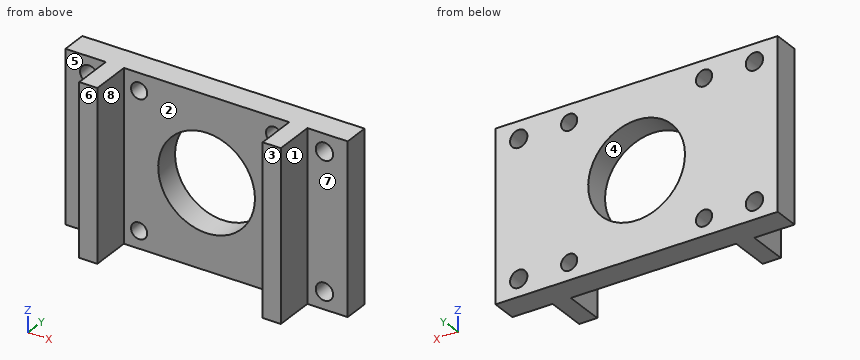
```python
from build123d import *

# Parameters (mm, degrees)
SKETCH1_W             = 70
SKETCH1_H             = 42
BOSS_EXTRUDE1_DEPTH   = 3.175
SKETCH3_W             = 4.5
SKETCH3_H             = 42
BOSS_EXTRUDE2_DEPTH   = 10
F_1_0MM_DOWEL_HOLE1_D = 4
F_1_0MM_DOWEL_HOLE2_D = 4.3
SKETCH4_R             = 12
CUT_EXTRUDE1_DEPTH    = 44.969563336


with BuildPart() as part:
    # Sketch1 → Boss-Extrude1 (new, symmetric)
    with BuildSketch(Plane(origin=(0, 0, 0), x_dir=(1, 0, 0), z_dir=(0, 1, 0))):
        Rectangle(SKETCH1_W, SKETCH1_H)
    extrude(amount=BOSS_EXTRUDE1_DEPTH, both=True)

    # Sketch3 → Boss-Extrude2 (add)
    with BuildSketch(Plane.XZ.offset(3.175)):
        with Locations((-22.75, 0)):
            Rectangle(SKETCH3_W, SKETCH3_H)
        with Locations((22.75, 0)):
            Rectangle(SKETCH3_W, SKETCH3_H)
    extrude(amount=BOSS_EXTRUDE2_DEPTH)

    # Ø1.0mm Dowel Hole1 (through all)
    with Locations(Plane(origin=(0, 3.175, 0), x_dir=(1, 0, 0), z_dir=(0, 1, 0))):
        with Locations((-16.73, 16.73), (16.73, 16.73), (16.73, -16.73), (-16.73, -16.73)):
            Hole(F_1_0MM_DOWEL_HOLE1_D / 2)

    # Ø1.0mm Dowel Hole2 (through all)
    with Locations(Plane(origin=(0, 3.175, 0), x_dir=(1, 0, 0), z_dir=(0, 1, 0))):
        with Locations((-29.23, 16.73), (-29.23, -16.73)):
            f_1_0mm_dowel_hole2 = Hole(F_1_0MM_DOWEL_HOLE2_D / 2)

    # Mirror1: Ø1.0mm Dowel Hole2 across plane
    add(f_1_0mm_dowel_hole2.mirror(Plane(origin=(0, 0, 0), x_dir=(0, 0, 1), z_dir=(1, 0, 0))), mode=Mode.SUBTRACT)

    # Sketch4 → Cut-Extrude1 (cut, through all)
    with BuildSketch(Plane(origin=(0, 3.175, 0), x_dir=(1, 0, 0), z_dir=(0, 1, 0))):
        with Locations(Location((0, 0, 0), (0, 0, 270))):
            Circle(SKETCH4_R)
    extrude(amount=-CUT_EXTRUDE1_DEPTH, mode=Mode.SUBTRACT)


solid = part.part
```
Check sheet for the modelled part. Datum: model origin and axes. Units: mm. Face numbers are marked on the shaded views. A direction names the side the tool comes from. Round coordinates to 2 decimals unless told otherwise and drop trailing zeros. Loops run counter-clockwise (first coordinate to the right, second up) from the corner with the lowest first, then second, coordinate; pieces in that order, holes last. Notation, with made-up numbers: M 51,47.5 L 81,47.5 A15 cw 81,56.5 Z; hole C 19,70 d11. An arc over 180 degrees is marked long. Answer as a JSON object with one key per item and string values.
1. Section check C-C (y = 1.5). State how many separate pieces and enclosed holes the cut face has, plus the area to 3 significant figures.
Reply:
{"separate pieces": "1", "enclosed holes": "9", "area": "2,380 mm²"}
2. Section check B-B (z = 16.73). Record the boundary of the cut face in (x, y) (3 decimals).
Reply:
{"outline": "M -35,-3.175 L -31.38,-3.175 L -31.38,3.175 L -35,3.175 Z; M -27.08,-3.175 L -25,-3.175 L -25,-13.175 L -20.5,-13.175 L -20.5,-3.175 L -18.73,-3.175 L -18.73,3.175 L -27.08,3.175 Z; M -14.73,-3.175 L 14.73,-3.175 L 14.73,3.175 L -14.73,3.175 Z; M 18.73,-3.175 L 20.5,-3.175 L 20.5,-13.175 L 25,-13.175 L 25,-3.175 L 27.08,-3.175 L 27.08,3.175 L 18.73,3.175 Z; M 31.38,-3.175 L 35,-3.175 L 35,3.175 L 31.38,3.175 Z"}
3. Section check A-A (x = -29.23). Record the boundary of the cut face in (y, z) (3 decimals), plus the area to 3 significant figures.
Reply:
{"outline": "M -3.175,-21 L 3.175,-21 L 3.175,-18.88 L -3.175,-18.88 Z; M -3.175,-14.58 L 3.175,-14.58 L 3.175,14.58 L -3.175,14.58 Z; M -3.175,18.88 L 3.175,18.88 L 3.175,21 L -3.175,21 Z", "area": "212 mm²"}
4. Access from +Z, -Z, +X, -X, +Y, -Y to the whole of each face (thin tool, end or side, straight path). Record for the marked faces 5, 6, 7 and 8.
Reply:
{"face 5": "+Z, -Z, -X, -Y", "face 6": "+Z, -Z, +X, -X, -Y", "face 7": "+Z, -Z, +X, -Y", "face 8": "+Z, -Z, -Y"}
5. Section check D-D (x = 0). Record the boundary of the cut face in (y, z) (3 decimals), plus the area to 3 significant figures.
Reply:
{"outline": "M -3.175,-21 L 3.175,-21 L 3.175,-12 L -3.175,-12 Z; M -3.175,12 L 3.175,12 L 3.175,21 L -3.175,21 Z", "area": "114 mm²"}
6. Gauge pin test, flat ends, axial feed: P1, Ø11, axis at x = 32.5, z = -5.5, coming from the -Y side (3 decimals); P2, Ø1, axis at y = -11, z = 16.5, coming from the +X side; P3, Ø3, axis at y = -8, z = 4, coming from the -X side. Record the tip position at first contact, or that the pin passes through.
Reply:
{"P1": "stops at y = -3.175", "P2": "stops at x = 25", "P3": "stops at x = -25"}
7. Mould release check, pull along X, two halves, no side actions. Record for the marked faces 1, 2, 3 and 4: pulls with the +X half, pulls with the -X half, needs draft (parallel to the pull), parting line crosses it, or undercut.
Reply:
{"face 1": "pulls with the +X half", "face 2": "undercut", "face 3": "needs draft", "face 4": "undercut"}
8. Scan lines: line 1 (Z direction, x = 29.23, y = 0.5); line 2 (Z direction, x = -16.73, y = -1); line 3 (X direction, y = -7, z = 0). Record each from-to range of solid material in increasing order.
Reply:
{"line 1": "z = -21 to -18.88, -14.58 to 14.58, 18.88 to 21", "line 2": "z = -21 to -18.73, -14.73 to 14.73, 18.73 to 21", "line 3": "x = -25 to -20.5, 20.5 to 25"}
